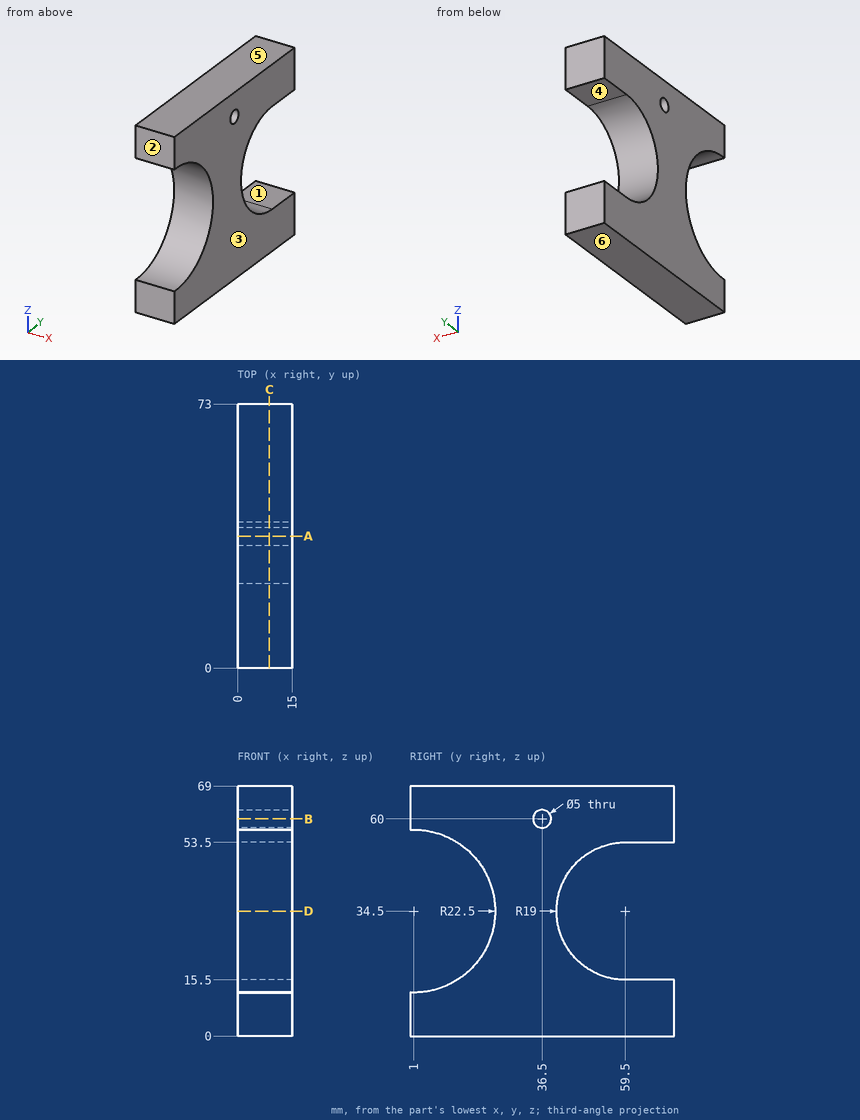
Geometry: see drawing. Coordinates: mm, zero at the bounding-box minimum. A direction names the side the tool comes from. Coordinates: 2 decimals unless noted, no trailing zeros. Write each loop counter-clockwise with the first axis right and the second up, starting at its lowest first coordinate (ties: lowest second). Pieces come first, ordered by that corner, then holes. Notation, with made-up numbers: M 60,60.25 L 113,60.25 A15 ccw 113,88.25 Z; hole C 61.5,-39 d9. An arc over 180 degrees is marked long. Use CSV: the item, a comma, the result in double quotes. Start each with the question number.
1. Cut plane B-B on z = 60. Return the cut outline in (x, y), plus the area to 3 significant figures.
2. Reachability of the marked faces 1 and 2 from +Z, -Z, +X, -X, +Y, -Y: full face, straight path, thin tool, end or side. Return the list, or none.
3. Cut plane A-A on y = 36.5. Return the cut outline in (x, z).
4. Cut plane C-C on x = 8.75. Return the cut outline in (y, z).
5. Ray query, probe 1 along Y at (x, z) = (7.5, 60); probe 2 along Z at (x, y) = (1, 70.5); probe 3 along Y at (x, z) = (6, 34). Return the intervals inside material, ascending.
6. Cut plane D-D on z = 34.5. Return the cut outline in (x, y).
7. First-contact query: P1, Ø4, axis at x = 13, z = 30.5, coming from the +Y side; P2, Ø2, axis at x = 3.5, z = 19.5, coming from the -Y side. Flat tips, straight axial feed; report the tip coordinate or a pass-through.
8. Mould query, pull axis Z, two halves, no side actions, for the marked faces 3, 4, 5 and 6. Classes: pulls with the +Z half, pulls with the -Z half, needs draft (parallel to the pull), parting line crosses it, or undercut.
Entries:
1,outline,"M 0,0 L 15,0 L 15,34 L 0,34 Z; M 0,39 L 15,39 L 15,73 L 0,73 Z"
1,area,"1,020 mm²"
2,face 1,"+X, -X, +Y"
2,face 2,"+Z, -Z, +X, -X, -Y"
3,outline,"M 0,0 L 15,0 L 15,57.5 L 0,57.5 Z; M 0,62.5 L 15,62.5 L 15,69 L 0,69 Z"
4,outline,"M 0,0 L 73,0 L 73,15.5 L 59.5,15.5 A19 cw 59.5,53.5 L 73,53.5 L 73,69 L 0,69 L 0,56.98 A22.5 cw long 0,12.02 Z; hole C 36.5,60 d5"
5,probe 1,"0 to 34, 39 to 73"
5,probe 2,"0 to 15.5, 53.5 to 69"
5,probe 3,"23.49 to 40.51"
6,outline,"M 0,23.5 L 15,23.5 L 15,40.5 L 0,40.5 Z"
7,P1,"y = 41.47"
7,P2,"y = 16.82"
8,face 3,"needs draft"
8,face 4,"undercut"
8,face 5,"pulls with the +Z half"
8,face 6,"pulls with the -Z half"
